Geometry check sheet. Reference: the model listing, model coordinates, mm. A direction names the side the tool comes from. Coordinates: 2 decimals unless noted, no trailing zeros. Loops run counter-clockwise (first coordinate to the right, second up) from the corner with the lowest first, then second, coordinate; pieces in that order, holes last. Notation, with made-up numbers: (42, 9) - (73, 9) arc R35 cw to (73, 46) - close; hole circle Ø6 at (19, 37). An arc over 180 degrees is marked (long way). Write item = value, one per line. Start each with the question number.
from build123d import *

# Parameters (mm, degrees)
F0_W     = 8.6
F0_H     = 2
F0_W_2   = 7.6
F0_H_2   = 1
F1_DEPTH = 5
F2_W     = 8.6
F2_H     = 3.75
F3_DEPTH = 1.25
F5_DEPTH = 8.601
F6_R     = 0.4


with BuildPart() as f1:
    # F0 (on Front) → F1 (new body)
    with BuildSketch(Plane.XZ):
        Rectangle(F0_W, F0_H)
        Rectangle(F0_W_2, F0_H_2, mode=Mode.SUBTRACT)
    extrude(amount=F1_DEPTH)

    # F2 (on face) → F3 (join)
    with BuildSketch(Plane.XZ.offset(5)):
        with Locations((0, 0.875)):
            Rectangle(F2_W, F2_H)
    extrude(amount=F3_DEPTH)

    # F4 (on face) → F5 (cut, through all)
    with BuildSketch(Plane.YZ.offset(4.3)):
        Polygon((-5, 1), (-5, 2.75), (-5.25, 1), align=None)
    extrude(amount=-F5_DEPTH, mode=Mode.SUBTRACT)

    # F6
    f6_edges = [f1.edges().sort_by_distance(p)[0] for p in [
        (0, -5.25, 1),
    ]]
    fillet(f6_edges, radius=F6_R)


solid = f1.part
(1) Sectioned sample at C-C on z = 0. Enter the section's corners in (x, y), plus the area to 4 significant figures.
(2) Tool access check on faces 4 (the face through (0.06, -5.09, 2.11)), 5 (the face through (0, -2, -0.5)), 6 (the face through (0, -6, 2.75)). Record the directions out of +Z, -Z, +X, -X, +Y, -Y that give a thin tool (end or side, any length) a straight path to the whole face; none if there is none.
(3) Scan lines: line 1 (Z direction, x = 0.5, y = -3.5); line 2 (X direction, y = -3.5, z = 0.35); line 3 (Y direction, x = -2.25, z = -0.05). Record each from-to range of solid material in increasing order.
(4) Draft check along X on faces 1 (the face through (0, -2, 1)), 2 (the face through (0, -2, 0.5)), 3 (the face through (4.3, -3, 0)). Enter one of: pulls with the +X half, pulls with the -X half, needs draft (parallel to the pull), parting line crosses it, or undercut.
(5) Depth check by flat-ended pin: pin 1 (0.8 mm diameter, centred on x = 1.5, z = 0, fed in from +Y). Enter the tip coordinate at first touch or a pass-through.
(6) Sectioned sample at D-D on z = 2.15. Enter the section's corners in (x, y).
(7) Sectioned sample at A-A on y = -1.25. Enter the section's corners in (x, z), plus the area to 3 significant figures.
(8) Sectioned sample at B-B on x = 0.25. Enter the section's corners in (y, z).
Working result:
q1.outline = (-4.3, -6.25) - (4.3, -6.25) - (4.3, 0) - (3.8, 0) - (3.8, -5) - (-3.8, -5) - (-3.8, 0) - (-4.3, 0) - close
q1.area = 15.75 mm2
q2.face_4 = +X, -X, +Y
q2.face_5 = +Y
q2.face_6 = +Z, +X, -X, +Y, -Y
q3.line_1 = -1 to -0.5, 0.5 to 1
q3.line_2 = -4.3 to -3.8, 3.8 to 4.3
q3.line_3 = -6.25 to -5
q4.face_1 = needs draft
q4.face_2 = undercut
q4.face_3 = pulls with the +X half
q5.pin_1 = -5
q6.outline = (-4.3, -6.25) - (4.3, -6.25) - (4.3, -5.09) - (-4.3, -5.09) - close
q7.outline = (-4.3, -1) - (4.3, -1) - (4.3, 1) - (-4.3, 1) - close; hole (-3.8, -0.5) - (3.8, -0.5) - (3.8, 0.5) - (-3.8, 0.5) - close
q7.area = 9.60 mm2
q8.outline = (-6.25, -1) - (0, -1) - (0, -0.5) - (-5, -0.5) - (-5, 0.5) - (0, 0.5) - (0, 1) - (-4.79, 1) arc R0.4 cw to (-5.18, 1.46) - (-5, 2.75) - (-6.25, 2.75) - close
